Verification items for this drawing (mm, ordinates from the low corner). A direction names the side the tool comes from. Round coordinates to 2 decimals unless told otherwise and drop trailing zeros. Order: outer loops, then holes, each group sorted by start corner. A loop starts at its lowest first (then second) coordinate and runs counter-clockwise, first axis right, second up. Notation, with made-up numbers: M 29.5,79 L 88.5,79 A32 ccw 88.5,117 Z; hole C 49.5,-11 d1. An arc over 180 degrees is marked long. Use CSV: the item, a comma, the result in double quotes. Start each with the question number.
Q1. Gauge pin test, flat ends, axial feed: pin 1 Ø3.5 at (y, z) = (12.5, 5.5) entering from -X (1 decimal); pin 2 Ø4 at (x, z) = (20.5, 8) entering from +Y; pin 3 Ø2 at (y, z) = (45.5, 2.5) entering from -X (1 decimal); pin 4 Ø2 at (x, y) = (55, 82) entering from -Z. Record the tip position at first contact, or that the pin passes through.
Q2. Scan lines: line 1 (Y direction, x = 50, z = 3.5); line 2 (X direction, y = 29, z = 2); line 3 (X direction, y = 53.5, z = 7.25) (1 decimal). Record each from-to range of solid material in increasing order.
Q3. Sectioned sample at B-B (y = 15). Enter the section's corners in (x, z).
Q4. Set-up check for the marked faces 5 and 6: record each of +Z, -Z, +X, -X, +Y, -Y from which the full face is reachable in a straight line by a thin tool's end or side.
Q5. Sectioned sample at C-C (z = 10.75). Enter the section's corners in (x, y), and give its area (3 significant figures).
Q6. Mould release check, pull along X, two halves, no side actions. Record for the marked faces 1, 2, 3 and 4: +X half, -X half, draft (parallel to the pull), parting line (faces both ways), or undercut.
Q7. Sectioned sample at A-A (x = 50). Enter the section's corners in (y, z).
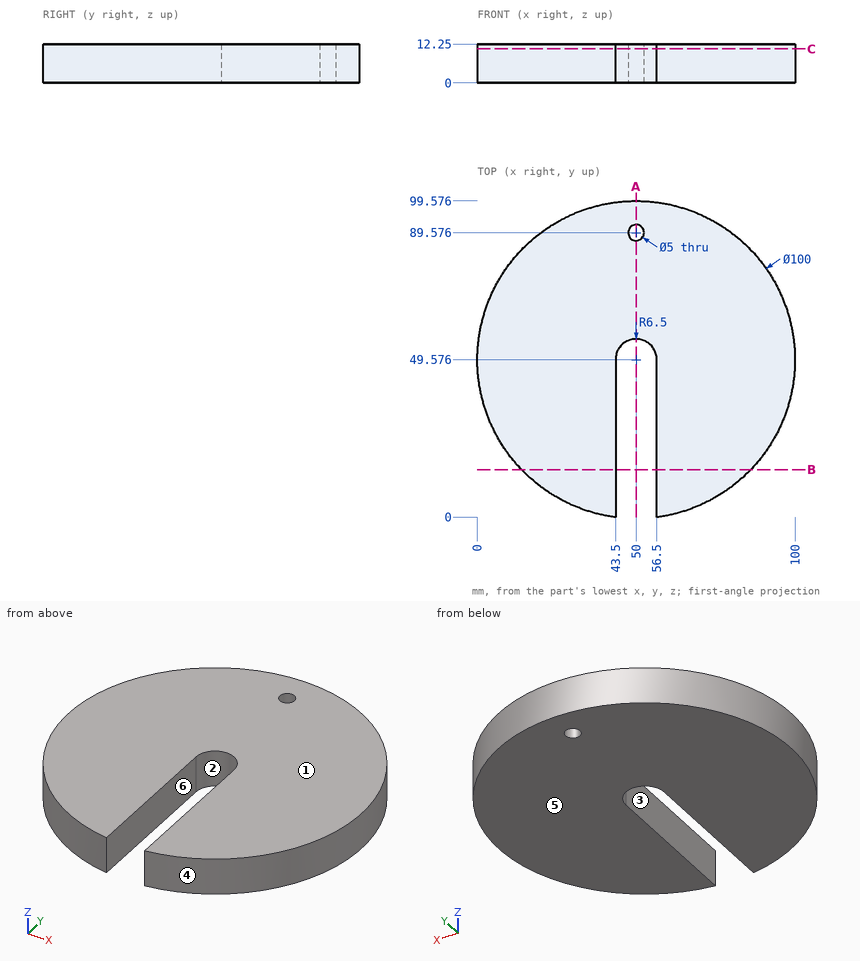
Verdict:
1,pin 1,"stops at x = 14.6"
1,pin 2,"stops at y = 91.33"
1,pin 3,"stops at x = 0.1"
1,pin 4,"stops at z = 0"
2,line 1,"y = 56.08 to 87.08, 92.08 to 99.58"
2,line 2,"x = 4.43 to 43.5, 56.5 to 95.57"
2,line 3,"x = 0.2 to 44.8, 55.2 to 99.8"
3,outline,"M 13.88,0 L 43.5,0 L 43.5,12.25 L 13.88,12.25 Z; M 56.5,0 L 86.12,0 L 86.12,12.25 L 56.5,12.25 Z"
4,face 5,"-Z, +X, -X, +Y, -Y"
4,face 6,"+Z, -Z, -Y"
5,outline,"M 43.5,0 L 43.5,49.58 A6.5 cw 56.5,49.58 L 56.5,0 A50 ccw long Z; hole C 50,89.58 d5"
5,area,"7,120 mm²"
6,face 1,"draft"
6,face 2,"undercut"
6,face 3,"undercut"
6,face 4,"parting line"
7,outline,"M 56.08,0 L 87.08,0 L 87.08,12.25 L 56.08,12.25 Z; M 92.08,0 L 99.58,0 L 99.58,12.25 L 92.08,12.25 Z"
